The model under review builds one solid part; all positions refer to its coordinate system, in mm. Face numbers are marked on the shaded views. A direction names the side the tool comes from. Round coordinates to 2 decimals unless told otherwise and drop trailing zeros. Return JSON: item names as keys, results as strings.
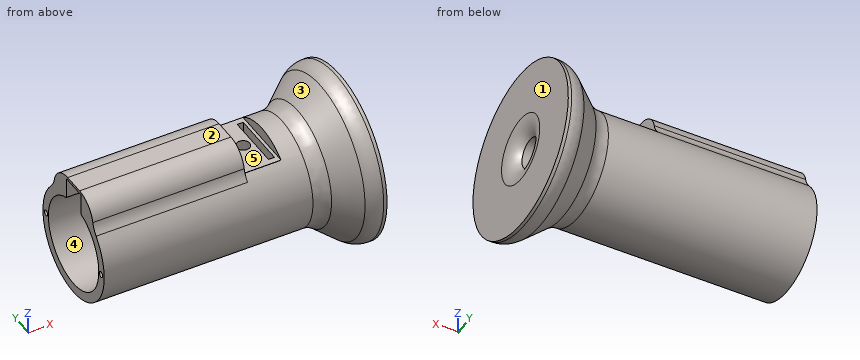
from build123d import *

# Parameters (mm, degrees)
SCHIZZO3_W                             = 9.243109639
SCHIZZO3_H                             = 30.902871456
TAGLIO_ESTRUSIONE2_DEPTH               = 78
SCHIZZO4_W                             = 15
SCHIZZO4_H                             = 28
ESTRUSIONE_ESTRUSIONE1_DEPTH           = 12
FORO_PER_VITE_M4_2_D                   = 37
FORO_PER_VITE_M4_2_DEPTH               = 60
FORO_PER_VITE_M5_1_D                   = 5.5
FORO_PER_VITE_M5_1_DEPTH               = 10
FORO_PER_VITE_M5_2_D                   = 5.5
FORO_PER_VITE_M5_2_DEPTH               = 10
FORO_PER_VITE_M2_2_D                   = 2.4
FORO_PER_VITE_M2_2_DEPTH               = 4
FORO_PER_VITE_M2_2_TIP                 = 0.721032743
SCHIZZO28_W                            = 62.660258955
SCHIZZO28_H                            = 27.779148216
ESTRUSIONE_ESTRUSIONE7_DEPTH           = 10
SCHIZZO29_W                            = 8.847921359
SCHIZZO29_H                            = 10.755513732
TAGLIO_ESTRUSIONE5_DEPTH               = 60
RACCORDO20_R                           = 10
RACCORDO21_R                           = 10
RACCORDO22_R                           = 10
RACCORDO24_R                           = 10
RACCORDO25_R                           = 10
RACCORDO26_R                           = 10
RACCORDO27_R                           = 10
SCHIZZO30_R                            = 6.061580104
TAGLIO_ESTRUSIONE6_DEPTH               = 23
SCHIZZO31_W                            = 2.5
SCHIZZO31_H                            = 23
TAGLIO_ESTRUSIONE7_DEPTH               = 23.75
FORO_SVASATO_PER_VITE_M3_1_D           = 3.4
FORO_SVASATO_PER_VITE_M3_1_CSINK_D     = 6.3
FORO_SVASATO_PER_VITE_M3_1_CSINK_ANGLE = 90


with BuildPart() as part:
    # Schizzo2 → Rivoluzione2 (revolve)
    with BuildSketch(Plane(origin=(0, 0, 0), x_dir=(1, 0, 0), z_dir=(0, 1, 0)), mode=Mode.PRIVATE) as rivoluzione2_sk:
        Polygon((-91.723538337, 22.5), (-91.723538337, 0), (14.335392963, 0), (14.335392963, 6.061580104), (18.276461663, 6.061580104), (18.276461663, 35), (13.276461663, 35), (-1.723538337, 22.5), align=None)
    revolve(rivoluzione2_sk.sketch.rotate(Axis((-119.689698016, 0, 0), (1, 0, 0)), 180), axis=Axis((-119.689698016, 0, 0), (1, 0, 0)))

    # Schizzo3 → Taglio-Estrusione2 (cut)
    with BuildSketch(Plane.ZY.offset(91.723538337)):
        with Locations((22.322677132, 0)):
            Rectangle(SCHIZZO3_W, SCHIZZO3_H)
    extrude(amount=-TAGLIO_ESTRUSIONE2_DEPTH, mode=Mode.SUBTRACT)

    # Schizzo4 → Estrusione-Estrusione1 (add)
    with BuildSketch(Plane.XY.offset(17.701122312)):
        with Locations((-21.563279382, 0)):
            Rectangle(SCHIZZO4_W, SCHIZZO4_H)
    extrude(amount=-ESTRUSIONE_ESTRUSIONE1_DEPTH)

    # Foro per Vite M4-2
    with Locations(Plane.ZY.offset(91.723538337)):
        with Locations((0, 0)):
            Hole(FORO_PER_VITE_M4_2_D / 2, depth=FORO_PER_VITE_M4_2_DEPTH)

    # Foro per Vite M5-1
    with Locations(Plane.XY.offset(17.701122312)):
        with Locations((-21.563279382, 0)):
            Hole(FORO_PER_VITE_M5_1_D / 2, depth=FORO_PER_VITE_M5_1_DEPTH)

    # Foro per Vite M5-2
    with Locations(Plane.ZY.offset(31.723538337)):
        with Locations((12.047310847, 0)):
            Hole(FORO_PER_VITE_M5_2_D / 2, depth=FORO_PER_VITE_M5_2_DEPTH)

    # Foro per Vite M2-2
    with Locations(Plane.ZY.offset(91.723538337)):
        with Locations((0, 20.2), (0, -20.2)):
            Hole(FORO_PER_VITE_M2_2_D / 2, depth=FORO_PER_VITE_M2_2_DEPTH)
            with Locations((0, 0, -(FORO_PER_VITE_M2_2_DEPTH + FORO_PER_VITE_M2_2_TIP / 2))):  # 118° drill point
                Cone(0, FORO_PER_VITE_M2_2_D / 2, FORO_PER_VITE_M2_2_TIP, mode=Mode.SUBTRACT)

    # Schizzo28 → Estrusione-Estrusione7 (add)
    with BuildSketch(Plane.XY.offset(17.701122312)):
        with Locations((-60.39340886, 0)):
            Rectangle(SCHIZZO28_W, SCHIZZO28_H)
    extrude(amount=ESTRUSIONE_ESTRUSIONE7_DEPTH)

    # Schizzo29 → Taglio-Estrusione5 (cut)
    with BuildSketch(Plane.ZY.offset(91.723538337)):
        with Locations((22.125082992, 0)):
            Rectangle(SCHIZZO29_W, SCHIZZO29_H)
    extrude(amount=-TAGLIO_ESTRUSIONE5_DEPTH, mode=Mode.SUBTRACT)

    # Raccordo20
    # the kernel refuses this fillet: 10 mm, written as the material it takes off along each edge
    with BuildSketch(Plane(origin=(18.276461663, 0, 0), x_dir=(0, 0, 1), z_dir=(0, 1, 0))) as raccordo20_piece_1:
        with BuildLine():
            CenterArc((14.017040588, -10), RACCORDO20_R, 90, 52.706861747)
            Line((6.061580104, -3.9410687), (5.902470894, -3.819890074))
            ThreePointArc((5.902470894, -3.819890074), (5.861580104, -1.97053435), (5.861580104, 0))
            Line((5.861580104, 0), (6.061580104, 0.2))
            Line((6.061580104, 0.2), (14.017040588, 0.2))
            Line((14.017040588, 0.2), (14.017040588, 0))
        make_face()
    revolve(axis=Axis((18.276461663, 0, 0), (1, 0, 0)), mode=Mode.SUBTRACT)

    # Raccordo21
    raccordo21_edges = [part.edges().sort_by_distance(p)[0] for p in [
        (13.276461663, 0, -35),
    ]]
    fillet(raccordo21_edges, radius=RACCORDO21_R)

    # Raccordo22
    raccordo22_edges = [part.edges().sort_by_distance(p)[0] for p in [
        (-1.723538337, 0, -22.5),
    ]]
    fillet(raccordo22_edges, radius=RACCORDO22_R)

    # Raccordo24
    # the kernel refuses this fillet: 10 mm, written as the material it adds along each edge
    with BuildSketch(Plane(origin=(-29.063279382, 13.889574108, 17.701122312), x_dir=(0, 0.7347199128018105, -0.6783705843655811), z_dir=(-1, 0, 0))) as raccordo24_piece_1:
        with BuildLine():
            CenterArc((4.407269799, -9.967842465), RACCORDO24_R, 94.596163378, 42.687391022)
            Line((-2.939929329, -3.184136621), (0, 0))
            ThreePointArc((0, 0), (1.802974009, -0.072354454), (3.605948017, 0))
        make_face()
    extrude(amount=62.660258955)

    # Raccordo25
    raccordo25_edges = [part.edges().sort_by_distance(p)[0] for p in [
        (-60.393408859, 13.889574108, 27.701122312),
    ]]
    fillet(raccordo25_edges, radius=RACCORDO25_R)

    # Raccordo26
    # the kernel refuses this fillet: 10 mm, written as the material it adds along each edge
    with BuildSketch(Plane(origin=(-29.063279382, -13.889574108, 17.701122312), x_dir=(0, -0.7347199128018104, -0.6783705843655813), z_dir=(-1, 0, 0))) as raccordo26_piece_1:
        with BuildLine():
            CenterArc((4.407269799, 9.967842465), RACCORDO26_R, 222.7164456, 42.687391022)
            Line((-2.939929329, 3.184136621), (0, 0))
            ThreePointArc((0, 0), (1.802974009, 0.072354454), (3.605948017, 0))
        make_face()
    extrude(amount=62.660258955)

    # Raccordo27
    raccordo27_edges = [part.edges().sort_by_distance(p)[0] for p in [
        (-60.393408859, -13.889574108, 27.701122312),
    ]]
    fillet(raccordo27_edges, radius=RACCORDO27_R)

    # Schizzo30 → Taglio-Estrusione6 (cut)
    with BuildSketch(Plane(origin=(14.335392963, 0, 0), x_dir=(0, 0, -1), z_dir=(1, 0, 0))):
        Circle(SCHIZZO30_R)
    extrude(amount=-TAGLIO_ESTRUSIONE6_DEPTH, mode=Mode.SUBTRACT)

    # Schizzo31 → Taglio-Estrusione7 (cut)
    with BuildSketch(Plane.XY.offset(17.701122312)):
        with Locations((-16.268538337, 0)):
            Rectangle(SCHIZZO31_W, SCHIZZO31_H)
    extrude(amount=-TAGLIO_ESTRUSIONE7_DEPTH, mode=Mode.SUBTRACT)

    # Foro svasato per Vite M3-1 (through all)
    with Locations(Plane(origin=(-8.664607037, 0, 0), x_dir=(0, 0, -1), z_dir=(1, 0, 0))):
        with Locations((0, 0)):
            CounterSinkHole(FORO_SVASATO_PER_VITE_M3_1_D / 2, FORO_SVASATO_PER_VITE_M3_1_CSINK_D / 2, counter_sink_angle=FORO_SVASATO_PER_VITE_M3_1_CSINK_ANGLE)


solid = part.part
(1) Add section A-A (y = 0). Give the number of separate pieces and of enclosed holes in the cut face, plus the area to 3 significant figures.
Filled in:
{"separate pieces": "4", "enclosed holes": "0", "area": "2,240 mm2"}
(2) Mouldability with a two-part tool opening along Y and no side actions: class the marked faces 3, 4 and 5 as released by +Y, released by -Y, zero draft, split by the parting line, or undercut.
Filled in:
{"face 3": "split by the parting line", "face 4": "undercut", "face 5": "zero draft"}
(3) Clearance check with flat-ended pins moving along their axes: pin 1 Ø4 at (x, y) = (-72, -13) entering from +Z; pin 2 Ø1.2 at (x, z) = (-15.5, 6) entering from -Y; pin 3 Ø1.4 at (y, z) = (20.2, 0) entering from -X. State where each tip first meets the part, or that it passes through.
Filled in:
{"pin 1": "stops at z = 25.18", "pin 2": "stops at y = -21.84", "pin 3": "stops at x = -87.42"}
(4) For the marked faces 1 and 2, list the 3-axis set-ups (+Z, -Z, +X, -X, +Y, -Y) from which the entire face can be reached by the end or side of a thin tool; tool diameter is ignored.
Filled in:
{"face 1": "+Z, -Z, +X, +Y, -Y", "face 2": "+Z, -X, +Y, -Y"}
(5) Wall thickness on line 1 (Y direction, x = -89, z = 0); line 2 (X direction, y = -1, z = -4.5); line 3 (X direction, y = 7.5, z = -16.5): over which ranges is each line inside the solid? List them lowest first.
Filled in:
{"line 1": "y = -22.5 to -21.4, -19 to -18.5, 18.5 to 19, 21.4 to 22.5", "line 2": "x = -31.72 to -17.52, -15.02 to -8.66", "line 3": "x = -31.72 to 18.28"}
